```python
from build123d import *

# Parameters (mm, degrees)
SKETCH1_R               = 3.6
SKETCH1_R_2             = 2.55
BOSS_EXTRUDE1_DEPTH     = 5
SKETCH2_R               = 6
SKETCH2_R_2             = 5.05
CUT_EXTRUDE1_DEPTH      = 2
SALIENTE_EXTRUIR1_DEPTH = 5
CROQUIS5_R              = 2.55
CORTAR_EXTRUIR2_DEPTH   = 6
CROQUIS6_R              = 1.55
CROQUIS6_W              = 6
CROQUIS6_H              = 4.2
CORTAR_EXTRUIR3_DEPTH   = 6
CORTAR_EXTRUIR4_DEPTH   = 6
CROQUIS8_R              = 4.625
CORTAR_EXTRUIR5_DEPTH   = 3.3


with BuildPart() as part:
    # Sketch1 → Boss-Extrude1 (new body)
    with BuildSketch(Plane(origin=(0, 0, 0), x_dir=(1, 0, 0), z_dir=(0, 1, 0))):
        with BuildLine():
            Line((20.365, -35), (-20.365, -35))
            ThreePointArc((-20.365, -35), (-23.642439931, -33.642439931), (-25, -30.365))
            Line((-25, -30.365), (-25, 30.365))
            ThreePointArc((-25, 30.365), (-23.642439931, 33.642439931), (-20.365, 35))
            Line((-20.365, 35), (20.365, 35))
            ThreePointArc((20.365, 35), (23.642439931, 33.642439931), (25, 30.365))
            Line((25, 30.365), (25, -30.365))
            ThreePointArc((25, -30.365), (23.642439931, -33.642439931), (20.365, -35))
        make_face()
        with Locations((-15, 25.95)):
            Circle(SKETCH1_R, mode=Mode.SUBTRACT)
        with Locations((15, 25.95)):
            Circle(SKETCH1_R, mode=Mode.SUBTRACT)
        with Locations((15, -25.95)):
            Circle(SKETCH1_R_2, mode=Mode.SUBTRACT)
        with Locations((-15, -25.95)):
            Circle(SKETCH1_R_2, mode=Mode.SUBTRACT)
    extrude(amount=BOSS_EXTRUDE1_DEPTH)

    # Sketch2 → Cut-Extrude1 (cut)
    with BuildSketch(Plane(origin=(0, 5, 0), x_dir=(1, 0, 0), z_dir=(0, 1, 0))):
        with Locations((-15, 25.95)):
            Circle(SKETCH2_R)
        with Locations((15, 25.95)):
            Circle(SKETCH2_R)
        with Locations((15, -25.95)):
            Circle(SKETCH2_R_2)
        with Locations((-15, -25.95)):
            Circle(SKETCH2_R_2)
    extrude(amount=-CUT_EXTRUDE1_DEPTH, mode=Mode.SUBTRACT)

    # Croquis3 → Saliente-Extruir1 (add)
    with BuildSketch(Plane(origin=(0, 5, 0), x_dir=(1, 0, 0), z_dir=(0, 1, 0))):
        with BuildLine():
            Line((-25, 30.365), (-25, 37))
            ThreePointArc((-25, 37), (-23.535533906, 40.535533906), (-20, 42))
            Line((-20, 42), (20, 42))
            ThreePointArc((20, 42), (23.535533906, 40.535533906), (25, 37))
            Line((25, 37), (25, 30.365))
            ThreePointArc((25, 30.365), (23.642439931, 33.642439931), (20.365, 35))
            Line((20.365, 35), (-20.365, 35))
            ThreePointArc((-20.365, 35), (-23.642439931, 33.642439931), (-25, 30.365))
        make_face()
        with BuildLine():
            Line((-20.365, -35), (20.365, -35))
            ThreePointArc((20.365, -35), (23.642439931, -33.642439931), (25, -30.365))
            Line((25, -30.365), (25, -37))
            ThreePointArc((25, -37), (23.535533906, -40.535533906), (20, -42))
            Line((20, -42), (-20, -42))
            ThreePointArc((-20, -42), (-23.535533906, -40.535533906), (-25, -37))
            Line((-25, -37), (-25, -30.365))
            ThreePointArc((-25, -30.365), (-23.642439931, -33.642439931), (-20.365, -35))
        make_face()
    extrude(amount=-SALIENTE_EXTRUIR1_DEPTH)

    # Croquis5 → Cortar-Extruir2 (cut, through all)
    with BuildSketch(Plane.XZ):
        with Locations((10, 1)):
            Circle(CROQUIS5_R)
        with Locations((-10, 1)):
            Circle(CROQUIS5_R)
    extrude(amount=-CORTAR_EXTRUIR2_DEPTH, mode=Mode.SUBTRACT)

    # Croquis6 → Cortar-Extruir3 (cut, through all)
    with BuildSketch(Plane(origin=(0, 5, 0), x_dir=(1, 0, 0), z_dir=(0, 1, 0))):
        with Locations((0, -37)):
            Circle(CROQUIS6_R)
        with Locations((-11, -37)):
            Rectangle(CROQUIS6_W, CROQUIS6_H)
        with Locations((11, -37)):
            Rectangle(CROQUIS6_W, CROQUIS6_H)
    cortar_extruir3 = extrude(amount=-CORTAR_EXTRUIR3_DEPTH, mode=Mode.SUBTRACT)

    # Croquis7 → Cortar-Extruir4 (cut, through all)
    with BuildSketch(Plane.XZ):
        with BuildLine():
            Line((-11.878679656, 39.1), (-10.121320344, 39.1))
            ThreePointArc((-10.121320344, 39.1), (-8.010608171, 39.110503119), (-7.979099854, 37))
            ThreePointArc((-7.979099854, 37), (-8.010608171, 34.889496881), (-10.121320344, 34.9))
            Line((-10.121320344, 34.9), (-11.878679656, 34.9))
            ThreePointArc((-11.878679656, 34.9), (-13.989391829, 34.889496881), (-14.020900146, 37))
            ThreePointArc((-14.020900146, 37), (-13.989391829, 39.110503119), (-11.878679656, 39.1))
        make_face()
        with BuildLine():
            Line((11.878679656, 34.9), (10.121320344, 34.9))
            ThreePointArc((10.121320344, 34.9), (8.010608171, 34.889496881), (7.979099854, 37))
            ThreePointArc((7.979099854, 37), (8.010608171, 39.110503119), (10.121320344, 39.1))
            Line((10.121320344, 39.1), (11.878679656, 39.1))
            ThreePointArc((11.878679656, 39.1), (13.989391829, 39.110503119), (14.020900146, 37))
            ThreePointArc((14.020900146, 37), (13.989391829, 34.889496881), (11.878679656, 34.9))
        make_face()
    cortar_extruir4 = extrude(amount=-CORTAR_EXTRUIR4_DEPTH, mode=Mode.SUBTRACT)

    # Croquis8 → Cortar-Extruir5 (cut)
    with BuildSketch(Plane.XZ):
        with Locations((-10, 1)):
            Circle(CROQUIS8_R)
        with Locations((10, 1)):
            Circle(CROQUIS8_R)
    extrude(amount=-CORTAR_EXTRUIR5_DEPTH, mode=Mode.SUBTRACT)

    # Simetría1: Cortar-Extruir3, Cortar-Extruir4 across plane
    add(cortar_extruir3.mirror(Plane.XY), mode=Mode.SUBTRACT)
    add(cortar_extruir4.mirror(Plane.XY), mode=Mode.SUBTRACT)


solid = part.part
```
Work out the finished part from the listing and answer in its coordinate system (mm). A direction names the side the tool comes from. Coordinates: 2 decimals unless noted, no trailing zeros. Write each loop counter-clockwise with the first axis right and the second up, starting at its lowest first coordinate (ties: lowest second). Pieces come first, ordered by that corner, then holes.
Q1. A cutting plane is placed at D-D, the plane y = 1.35. State how many separate pieces and enclosed holes the cut face has, then the cut area to 3 significant figures.
Q2. A cutting plane is placed at C-C, the plane z = 25.95. Give the vertices of the cut face in (x, y), then the cut area to 3 significant figures.
Q3. Find the intervals of material crossed by line 1 (X direction, y = 4.15, z = -25.95); line 2 (Z direction, x = 15, y = 1.2); line 3 (Z direction, x = -15, y = 3.9), in increasing order.
Q4. A cutting plane is placed at A-A, the plane z = 1. Give the vertices of the cut face in (x, y) (3 decimals), then the cut area to 3 significant figures.
Q5. Which of the six approach directions +Z, -Z, +X, -X, +Y, -Y give full straight-line access (tool end or side, diameter ignored) to faces 1 (the face through (0, 0, -1)), 2 (the face through (14.41, 1.63, 2.39)), 3 (the face through (18.226, 4.014, -31.009)), 4 (the face through (24, 3, 40)), 5 (the face through (-11, 3, 34.9))?
Q6. Each of these flat-tipped pins is pushed along its axis until it touches: pin 1 Ø6 at (x, z) = (12.5, -27.5) entering from +Y; pin 2 Ø7.5 at (x, z) = (10, 1) entering from -Y. Where does it stop, or does it pass through?
Q7. Determine the mould class of faces 6 (the face through (25, 3, -1)), 7 (the face through (0, 3, 42)), 8 (the face through (-5.728, 1.627, -0.771)) for opening direction Z: released by +Z, released by -Z, zero draft, split by the parting line, or undercut.
Q8. A cutting plane is placed at B-B, the plane x = 0. Give the vertices of the cut face in (y, z).
Findings below:
1. separate pieces: 1
1. enclosed holes: 12
1. area: 3,790 mm2
2. outline: (-25, 0) - (-17.55, 0) - (-17.55, 3) - (-20.05, 3) - (-20.05, 5) - (-25, 5) - close; (-12.45, 0) - (12.45, 0) - (12.45, 3) - (9.95, 3) - (9.95, 5) - (-9.95, 5) - (-9.95, 3) - (-12.45, 3) - close; (17.55, 0) - (25, 0) - (25, 5) - (20.05, 5) - (20.05, 3) - (17.55, 3) - close
2. area: 179 mm2
3. line 1: x = -25 to -21, -9 to 9, 21 to 25
3. line 2: z = -42 to -29.55, -22.35 to 23.4, 28.5 to 42
3. line 3: z = -42 to -31.95, -19.95 to 20.9, 31 to 42
4. outline: (-25, 0) - (-14.625, 0) - (-14.625, 3.3) - (-12.55, 3.3) - (-12.55, 5) - (-25, 5) - close; (-7.45, 3.3) - (-5.375, 3.3) - (-5.375, 0) - (5.375, 0) - (5.375, 3.3) - (7.45, 3.3) - (7.45, 5) - (-7.45, 5) - close; (12.55, 3.3) - (14.625, 3.3) - (14.625, 0) - (25, 0) - (25, 5) - (12.55, 5) - close
4. area: 172 mm2
5. face 1: +Z, -Z, +X, -X, -Y
5. face 2: -Y
5. face 3: +Y
5. face 4: +Z, +X, +Y, -Y
5. face 5: +Y, -Y
6. pin 1: stops at y = 3
6. pin 2: stops at y = 3.3
7. face 6: zero draft
7. face 7: released by +Z
7. face 8: undercut
8. outline: (0, -42) - (5, -42) - (5, -38.55) - (0, -38.55) - close; (0, -35.45) - (5, -35.45) - (5, 35.45) - (0, 35.45) - close; (0, 38.55) - (5, 38.55) - (5, 42) - (0, 42) - close
